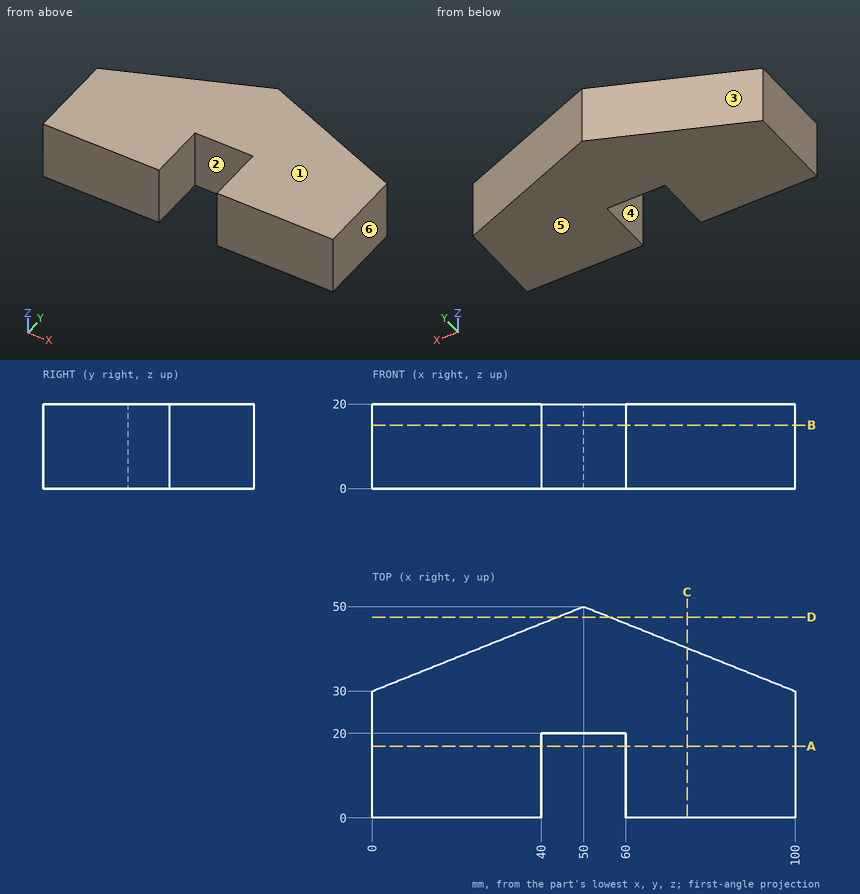
Input: dimensioned drawing with shaded views. Units: mm. Origin: part minimum x, y, z. A direction names the side the tool comes from. Round coordinates to 2 decimals unless told otherwise and drop trailing zeros. Loops run counter-clockwise (first coordinate to the right, second up) from the corner with the lowest first, then second, coordinate; pieces in that order, holes last. Notation, with made-up numbers: M 55,53.5 L 96,53.5 A23 cw 96,78.5 Z; hole C 32,43 d11. An arc over 180 degrees is marked long. Answer in a Markdown table with one row per item. Add a question column.
1. Set-up query: the marked faces 1 and 2. Return all of +Z, -Z, +X, -X, +Y, -Y with unobstructed straight access to the full face (end or side cutting, diameter ignored); none if empty.
2. Section A-A (y = 17). Output: boundary loops of the cut face in (x, z).
3. Contact query for flat-ended pins moving along their axis: pin 1 (6 mm diameter, centred on x = 68.5, y = 26.5, fed in from -Z); pin 2 (1 mm diameter, centred on x = 48.5, z = 14, fed in from -Y). Output: stop coordinate, or through.
4. Ray query, probe 1 along X at (y, z) = (6, 5); probe 2 along Y at (x, z) = (96.5, 7.5); probe 3 along Y at (x, z) = (6.5, 5.25). Return the intervals inside material, ascending.
5. Mould query, pull axis X, two halves, no side actions, for the marked faces 3, 4, 5 and 6. Classes: released by +X, released by -X, zero draft, split by the parting line, or undercut.
6. Section C-C (x = 74.5). Output: boundary loops of the cut face in (y, z).
7. Section B-B (z = 15). Output: boundary loops of the cut face in (x, y).
8. Section D-D (y = 47.5). Output: boundary loops of the cut face in (x, z).
Values follow:
| question | item | result |
|---|---|---|
| 1 | face 1 | +Z, +X, -X, +Y, -Y |
| 1 | face 2 | +Z, -Z, -Y |
| 2 | outline | M 0,0 L 40,0 L 40,20 L 0,20 Z; M 60,0 L 100,0 L 100,20 L 60,20 Z |
| 3 | pin 1 | z = 0 |
| 3 | pin 2 | y = 20 |
| 4 | probe 1 | 0 to 40, 60 to 100 |
| 4 | probe 2 | 0 to 31.4 |
| 4 | probe 3 | 0 to 32.6 |
| 5 | face 3 | released by -X |
| 5 | face 4 | undercut |
| 5 | face 5 | zero draft |
| 5 | face 6 | released by +X |
| 6 | outline | M 0,0 L 40.2,0 L 40.2,20 L 0,20 Z |
| 7 | outline | M 0,0 L 40,0 L 40,20 L 60,20 L 60,0 L 100,0 L 100,30 L 50,50 L 0,30 Z |
| 8 | outline | M 43.75,0 L 56.25,0 L 56.25,20 L 43.75,20 Z |
